Can you work these out from the drawing? Everything is in mm from the part's minimum corner. Round coordinates to 2 decimals unless told otherwise and drop trailing zeros. Write each loop counter-clockwise with the first axis right and the second up, starting at its lowest first coordinate (ties: lowest second). Pieces come first, ordered by that corner, then holes. Notation, with made-up numbers: (21, 64) -> (53, 64) arc R23 ccw to (53, 87) -> close; hole circle Ø1 at (69, -6.5). An arc over 180 degrees is marked (long way). Write item = value, one per line. Start each with the question number.
1) I'm going to push flat-ended pins straight in: pin 1 (2 mm diameter, centred on x = 403.5, y = 150.5, fed in from +Z); pin 2 (25 mm diameter, centred on x = 14.5, y = 141, fed in from +Z); pin 3 (15 mm diameter, centred on x = 780.5, y = 288.5, fed in from -Z). Where does each tip first touch, or does it pass through?
2) If I drill on line 1 (X direction, y = 480, z = 833); line 2 (Z direction, x = 512.5, y = 175); line 3 (Y direction, x = 766.5, z = 637.5), over which ranges is the centre line in solid material (lowest first)?
3) Imagine slicing it at D-D, the plane x = 265.5. Please give me the cut outline in (y, z).
4) Imagine slicing it at C-C, the plane z = 363. Please give me the cut outline in (x, y), then the cut area to 3 significant figures.
5) Imagine slicing it at B-B, the plane y = 334. Please give me the cut outline in (x, z), then the cut area to 3 significant figures.
6) Imagine slicing it at A-A, the plane z = 793.5. Please give me the cut outline in (x, y), then the cut area to 3 significant figures.
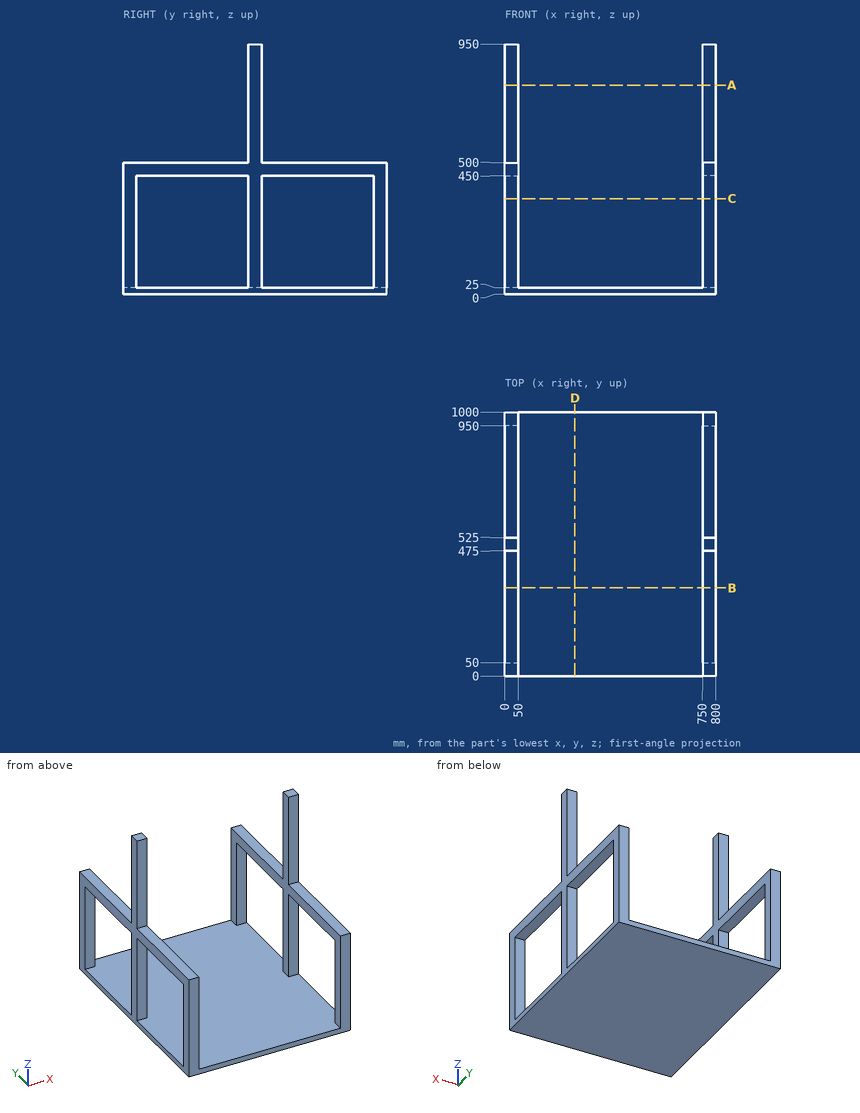
Reported:
q1.pin_1 = 25
q1.pin_2 = 500
q1.pin_3 = 0
q2.line_1 = 0 to 50, 750 to 800
q2.line_2 = 0 to 25
q2.line_3 = 475 to 525
q3.outline = (0, 0) -> (1000, 0) -> (1000, 25) -> (0, 25) -> close
q4.outline = (0, 0) -> (50, 0) -> (50, 50) -> (0, 50) -> close; (0, 475) -> (50, 475) -> (50, 525) -> (0, 525) -> close; (0, 950) -> (50, 950) -> (50, 1000) -> (0, 1000) -> close; (750, 0) -> (800, 0) -> (800, 50) -> (750, 50) -> close; (750, 475) -> (800, 475) -> (800, 525) -> (750, 525) -> close; (750, 950) -> (800, 950) -> (800, 1000) -> (750, 1000) -> close
q4.area = 15,000 mm²
q5.outline = (0, 0) -> (800, 0) -> (800, 25) -> (0, 25) -> close; (0, 450) -> (50, 450) -> (50, 500) -> (0, 500) -> close; (750, 450) -> (800, 450) -> (800, 500) -> (750, 500) -> close
q5.area = 25,000 mm²
q6.outline = (0, 475) -> (50, 475) -> (50, 525) -> (0, 525) -> close; (750, 475) -> (800, 475) -> (800, 525) -> (750, 525) -> close
q6.area = 5,000 mm²
